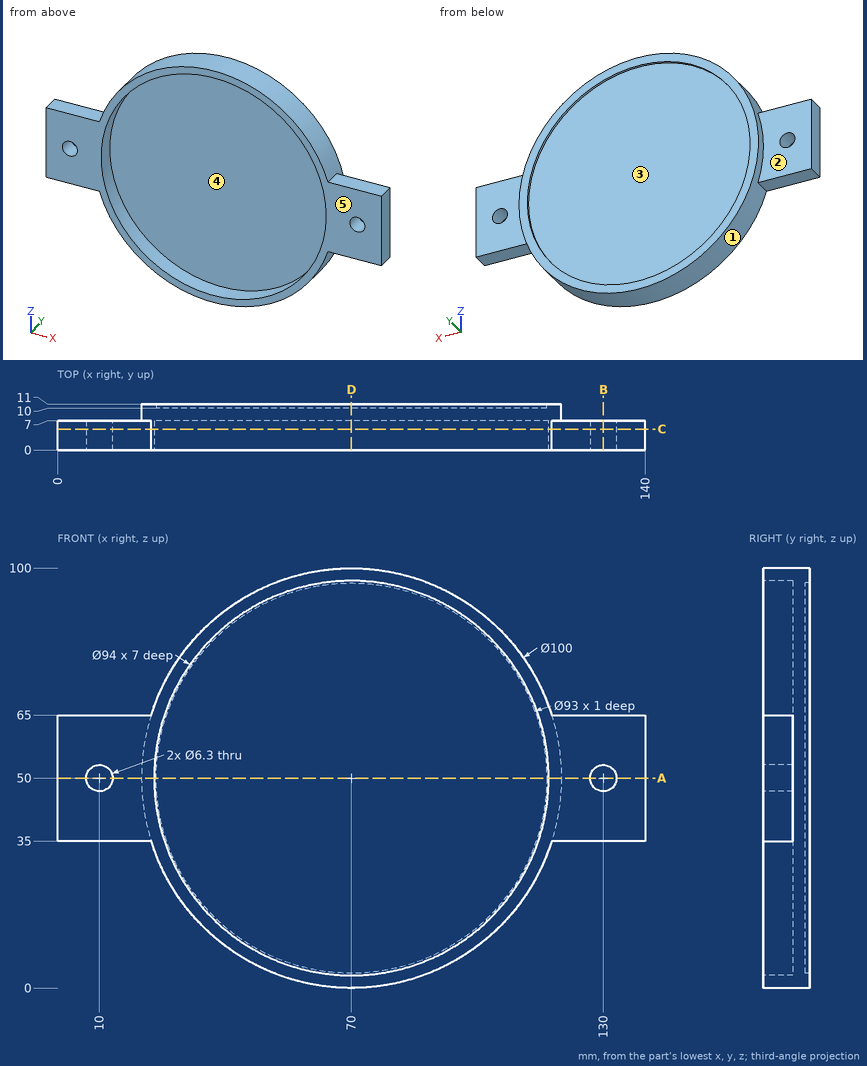
Can you work these out from the drawing? Everything is in mm from the part's minimum corner. A direction names the side the tool comes from. Give positions to 0.01 mm unless a question says otherwise; leave off trailing zeros. Loops run counter-clockwise (first coordinate to the right, second up) from the corner with the lowest first, then second, coordinate; pieces in that order, holes last. Notation, with made-up numbers: (-16, 46) -> (5, 46) arc R21 ccw to (5, 60) -> close; hole circle Ø10 at (22, 43.5). An arc over 180 degrees is marked (long way). Return JSON: item names as keys, results as strings.
Q1. I want a section at D-D, the plane x = 70. List the corners of the cut face in (y, z) for me, then the cut area to 3 significant figures.
Checks:
{"outline": "(0, 0) -> (11, 0) -> (11, 3.5) -> (10, 3.5) -> (10, 96.5) -> (11, 96.5) -> (11, 100) -> (0, 100) -> (0, 97) -> (7, 97) -> (7, 3) -> (0, 3) -> close", "area": "349 mm2"}
Q2. For pin 1 Ø2 at (x, y) = (133, 2) entering from -Z; pin 2 Ø8 at (x, z) = (66, 74) entering from -Y; pin 3 Ø2 at (x, y) = (97.5, 3) entering from +Z; pin 4 Ø24.5 at (x, z) = (130, 43.5) entering from +Y, each with a flat end and sliding along its axis, tell me the tip position at first contact or that it passes through.
Checks:
{"pin 1": "stops at z = 35", "pin 2": "stops at y = 7", "pin 3": "stops at z = 92.4", "pin 4": "stops at y = 11"}
Q3. On a 3-axis mill with a long thin cutter (end or side, diameter ignored), from which of +Z, -Z, +X, -X, +Y, -Y can I reach the whole of each face in a straight line? I mean the marked faces 4 and 5. Say none if no direction works.
Checks:
{"face 4": "-Y", "face 5": "+Z, -Z, +X, -X, -Y"}
Q4. I want a section at B-B, the plane x = 130. List the corners of the cut face in (y, z) for me.
Checks:
{"outline": "(0, 35) -> (7, 35) -> (7, 46.85) -> (0, 46.85) -> close; (0, 53.15) -> (7, 53.15) -> (7, 65) -> (0, 65) -> close"}
Q5. I want a section at C-C, the plane y = 5. List the corners of the cut face in (x, z) for me, then the cut area to 3 significant figures.
Checks:
{"outline": "(0, 35) -> (22.3, 35) arc R50 ccw to (117.7, 35) -> (140, 35) -> (140, 65) -> (117.7, 65) arc R50 ccw to (22.3, 65) -> (0, 65) -> close; hole circle Ø6.3 at (10, 50); hole circle Ø94 at (70, 50); hole circle Ø6.3 at (130, 50)", "area": "2,100 mm2"}
Q6. I need wall thicknesses on probe 1 along Z at (x, y) = (130, 1.5); probe 2 along Z at (x, y) = (70, 2.5); probe 3 along Y at (x, z) = (85, 90). Which ranges of each line are inside material? Lowest first, please.
Checks:
{"probe 1": "z = 35 to 46.85, 53.15 to 65", "probe 2": "z = 0 to 3, 97 to 100", "probe 3": "y = 7 to 10"}
Q7. I want a section at A-A, the plane z = 50. List the corners of the cut face in (x, y) for me.
Checks:
{"outline": "(0, 0) -> (6.85, 0) -> (6.85, 7) -> (0, 7) -> close; (13.15, 0) -> (23, 0) -> (23, 7) -> (117, 7) -> (117, 0) -> (126.85, 0) -> (126.85, 7) -> (120, 7) -> (120, 11) -> (116.5, 11) -> (116.5, 10) -> (23.5, 10) -> (23.5, 11) -> (20, 11) -> (20, 7) -> (13.15, 7) -> close; (133.15, 0) -> (140, 0) -> (140, 7) -> (133.15, 7) -> close"}
Q8. We'd pull the mould along Z, two halves only. Please class the marked faces 1, 2 and 3: released by +Z, released by -Z, zero draft, split by the parting line, or undercut.
Checks:
{"face 1": "split by the parting line", "face 2": "zero draft", "face 3": "undercut"}
